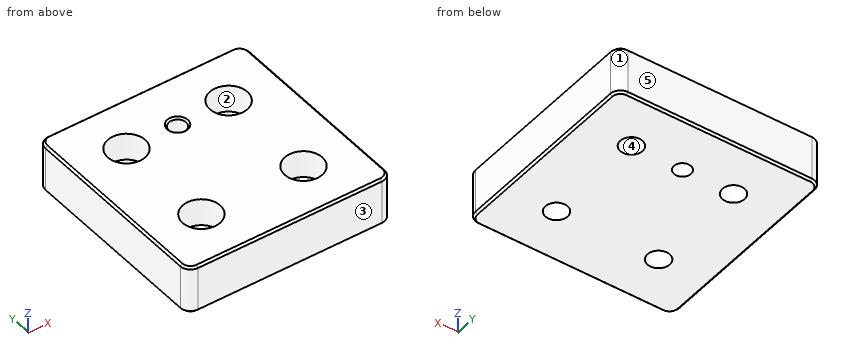
from build123d import *

# Parameters (mm, degrees)
SKETCH1_W                                           = 60
SKETCH1_H                                           = 60
BOSS_EXTRUDE1_DEPTH                                 = 14
CBORE_FOR_M6_HEX_SOCKET_HEAD_CAP_SCREW1_D           = 6.5
CBORE_FOR_M6_HEX_SOCKET_HEAD_CAP_SCREW1_CBORE_D     = 11
CBORE_FOR_M6_HEX_SOCKET_HEAD_CAP_SCREW1_CBORE_DEPTH = 8
M6_TAPPED_HOLE1_D                                   = 5
M6_TAPPED_HOLE1_CSINK_D                             = 6.05
M6_TAPPED_HOLE1_CSINK_ANGLE                         = 90
FILLET1_R                                           = 3
CHAMFER1_SIZE                                       = 0.6


with BuildPart() as part:
    # Sketch1 → Boss-Extrude1 (new body)
    with BuildSketch(Plane.XY):
        Rectangle(SKETCH1_W, SKETCH1_H)
    extrude(amount=BOSS_EXTRUDE1_DEPTH)

    # CBORE for M6 Hex Socket Head Cap Screw1 (through all)
    with Locations(Plane.XY.offset(14)):
        with Locations((-15, 15), (15, 15), (15, -15), (-15, -15)):
            CounterBoreHole(CBORE_FOR_M6_HEX_SOCKET_HEAD_CAP_SCREW1_D / 2, CBORE_FOR_M6_HEX_SOCKET_HEAD_CAP_SCREW1_CBORE_D / 2, CBORE_FOR_M6_HEX_SOCKET_HEAD_CAP_SCREW1_CBORE_DEPTH)

    # M6 Tapped Hole1 (through all)
    with Locations(Plane.XY.offset(14)):
        with Locations((0, 15)):
            CounterSinkHole(M6_TAPPED_HOLE1_D / 2, M6_TAPPED_HOLE1_CSINK_D / 2, counter_sink_angle=M6_TAPPED_HOLE1_CSINK_ANGLE)

    # Fillet1
    fillet1_edges = [part.edges().sort_by_distance(p)[0] for p in [
        (-30, 30, 7),
        (30, 30, 7),
        (30, -30, 7),
        (-30, -30, 7),
    ]]
    fillet(fillet1_edges, radius=FILLET1_R)

    # Chamfer1
    chamfer1_edges = [part.edges().sort_by_distance(p)[0] for p in [
        (-30, 0, 0),
        (-30, 0, 14),
        (0, 30, 0),
        (30, 0, 0),
        (0, -30, 0),
        (-29.121320344, -29.121320344, 0),
        (29.121320344, -29.121320344, 0),
        (29.121320344, 29.121320344, 0),
        (-29.121320344, 29.121320344, 0),
        (0, 30, 14),
        (0, -30, 14),
        (30, 0, 14),
        (-29.121320344, -29.121320344, 14),
        (29.121320344, -29.121320344, 14),
        (29.121320344, 29.121320344, 14),
        (-29.121320344, 29.121320344, 14),
    ]]
    chamfer(chamfer1_edges, length=CHAMFER1_SIZE)


solid = part.part
Geometry check sheet. Reference: the model listing, model coordinates, mm. Face numbers are marked on the shaded views. A direction names the side the tool comes from. Give positions to 0.01 mm unless a question says otherwise; leave off trailing zeros. Write each loop counter-clockwise with the first axis right and the second up, starting at its lowest first coordinate (ties: lowest second). Pieces come first, ordered by that corner, then holes.
1) Cross-section at C-C (z = 2). Record the boundary of the cut face in (x, y), plus the area to 3 significant figures.
Values follow:
outline: (-30, -27) arc R3 ccw to (-27, -30) - (27, -30) arc R3 ccw to (30, -27) - (30, 27) arc R3 ccw to (27, 30) - (-27, 30) arc R3 ccw to (-30, 27) - close; hole circle Ø6.5 at (-15, -15); hole circle Ø6.5 at (-15, 15); hole circle Ø5 at (0, 15); hole circle Ø6.5 at (15, -15); hole circle Ø6.5 at (15, 15)
area: 3,440 mm2
2) Go/stop test with flat-tipped pins: pin 1 Ø3.5 at (x, y) = (-17, 14) entering from +Z; pin 2 Ø5 at (x, y) = (-15, -15) entering from +Z. Record where each tip stops, or that it passes through.
Values follow:
pin 1: stops at z = 6
pin 2: passes through
3) Thickness scan on line 1 (Y direction, x = -15, z = 12.25); line 2 (Y direction, x = 15, z = 4.75); line 3 (X direction, y = 12, z = 9). Record the ranges inside material, lowest first.
Values follow:
line 1: y = -30 to -20.5, -9.5 to 9.5, 20.5 to 30
line 2: y = -30 to -18.25, -11.75 to 11.75, 18.25 to 30
line 3: x = -30 to -19.61, -10.39 to 10.39, 19.61 to 30
4) Cross-section at A-A (x = 0). Record the boundary of the cut face in (y, z) (3 decimals).
Values follow:
outline: (-30, 0.6) - (-29.4, 0) - (12.5, 0) - (12.5, 13.475) - (11.975, 14) - (-29.4, 14) - (-30, 13.4) - close; (17.5, 0) - (29.4, 0) - (30, 0.6) - (30, 13.4) - (29.4, 14) - (18.025, 14) - (17.5, 13.475) - close
5) Release check for a two-part mould opening along Y. For the marked faces 3, 4 and 5 record: released by +Y, released by -Y, zero draft, split by the parting line, or undercut.
Values follow:
face 3: released by -Y
face 4: undercut
face 5: released by +Y
6) Cross-section at B-B (y = -15). Record the boundary of the cut face in (x, z), plus the area to 3 significant figures.
Values follow:
outline: (-30, 0.6) - (-29.4, 0) - (-18.25, 0) - (-18.25, 6) - (-20.5, 6) - (-20.5, 14) - (-29.4, 14) - (-30, 13.4) - close; (-11.75, 0) - (11.75, 0) - (11.75, 6) - (9.5, 6) - (9.5, 14) - (-9.5, 14) - (-9.5, 6) - (-11.75, 6) - close; (18.25, 0) - (29.4, 0) - (30, 0.6) - (30, 13.4) - (29.4, 14) - (20.5, 14) - (20.5, 6) - (18.25, 6) - close
area: 585 mm2
7) Set-up check for the marked faces 1 and 2: record each of +Z, -Z, +X, -X, +Y, -Y from which the full face is reachable in a straight line by a thin tool's end or side.
Values follow:
face 1: +Z, -Z, +X, +Y
face 2: +Z
